Model file for the job. Use its own axes, mm. A direction names the side the tool comes from. Round coordinates to 2 decimals unless told otherwise and drop trailing zeros. Loops run counter-clockwise (first coordinate to the right, second up) from the corner with the lowest first, then second, coordinate; pieces in that order, holes last. Notation, with made-up numbers: (-14.5, 58.5) -> (-3.5, 58.5) arc R20 cw to (-3.5, 91.5) -> close; hole circle Ø10 at (-36.75, 65.5). An arc over 180 degrees is marked (long way). Use a Markdown table: item, result.
from build123d import *

# Parameters (mm, degrees)
SKETCH1_W                         = 152.4
SKETCH1_H                         = 88.9
BASE_FLANGE1_DEPTH                = 1.29032
EDGE_FLANGE1_STRIP_W              = 5.85978
EDGE_FLANGE1_STRIP_H              = 1.29032
EDGE_FLANGE1_STRIP_CUT_DEPTH      = 88.9
EDGE_FLANGE1_STRIP_2_W            = 5.85978
EDGE_FLANGE1_STRIP_2_H            = 1.29032
EDGE_FLANGE1_STRIP_CUT_2_DEPTH    = 88.9
EDGE_FLANGE1_DEPTH                = 88.9
EDGE_FLANGE1_BEND_DEPTH           = 88.9
F_4_22MM_HOLE_FOR_M3_CLINCH_NUT_D = 4.22
BREAK_CORNER1_START               = -77.68082
BREAK_CORNER1_DEPTH               = 155.36164
CUT_THICKEN1_START                = 41.91
CUT_THICKEN1_OUTLINE_W            = 0.127
CUT_THICKEN1_OUTLINE_H            = 1.29032
CUT_THICKEN1_DEPTH                = 2.54
CUT_THICKEN2_START                = 41.91
CUT_THICKEN2_OUTLINE_W            = 0.127
CUT_THICKEN2_OUTLINE_H            = 1.29032
CUT_THICKEN2_DEPTH                = 2.54
MIRROR7_START                     = 41.91
MIRROR7_COPY_1_SKETCH_W           = 0.127
MIRROR7_COPY_1_SKETCH_H           = 1.29032
MIRROR7_COPY_1_DEPTH              = 2.54
MIRROR7_COPY_2_SKETCH_W           = 0.127
MIRROR7_COPY_2_SKETCH_H           = 1.29032
MIRROR7_COPY_2_DEPTH              = 2.54
MOVE_FACE1_BY                     = 1.27
MOVE_FACE1_2_BY                   = 1.27
MOVE_FACE1_3_BY                   = 1.27
MOVE_FACE1_4_BY                   = 1.27
EDGE_FLANGE2_STRIP_W              = 5.66928
EDGE_FLANGE2_STRIP_H              = 1.29032
EDGE_FLANGE2_STRIP_CUT_DEPTH      = 2.54
EDGE_FLANGE2_STRIP_2_W            = 5.66928
EDGE_FLANGE2_STRIP_2_H            = 1.29032
EDGE_FLANGE2_STRIP_CUT_2_DEPTH    = 2.54
EDGE_FLANGE2_STRIP_3_W            = 5.66928
EDGE_FLANGE2_STRIP_3_H            = 1.29032
EDGE_FLANGE2_STRIP_CUT_3_DEPTH    = 2.54
EDGE_FLANGE2_STRIP_4_W            = 5.66928
EDGE_FLANGE2_STRIP_4_H            = 1.29032
EDGE_FLANGE2_STRIP_CUT_4_DEPTH    = 2.54
EDGE_FLANGE2_DEPTH                = 2.54
EDGE_FLANGE2_BEND_DEPTH           = 2.54
EDGE_FLANGE2_BEND_2_DEPTH         = 2.54
EDGE_FLANGE2_BEND_3_DEPTH         = 2.54


# Read off the part's stored shape, not the designer's step: Break-Corner1, Cut-Thicken1, Cut-Thicken2
# Sheet-metal steps are written as plain solids
with BuildPart() as part:
    # Sketch1 → Base-Flange1 (new body)
    with BuildSketch(Plane.XY):
        Rectangle(SKETCH1_W, SKETCH1_H)
    extrude(amount=-BASE_FLANGE1_DEPTH)

    # Edge-Flange1 strip (across the edge) → Edge-Flange1 strip cut (cut)
    with BuildSketch(Plane(origin=(-76.3905, -44.45, -1.29032), x_dir=(1, 0, 0), z_dir=(0, 1, 0))):
        with Locations((-2.67589, -0.64516)):
            Rectangle(EDGE_FLANGE1_STRIP_W, EDGE_FLANGE1_STRIP_H)
    extrude(amount=EDGE_FLANGE1_STRIP_CUT_DEPTH, mode=Mode.SUBTRACT)

    # Edge-Flange1 strip 2 (across the edge) → Edge-Flange1 strip cut 2 (cut)
    with BuildSketch(Plane(origin=(76.3905, 44.45, -1.29032), x_dir=(-1, 0, 0), z_dir=(0, -1, 0))):
        with Locations((-2.67589, -0.64516)):
            Rectangle(EDGE_FLANGE1_STRIP_2_W, EDGE_FLANGE1_STRIP_2_H)
    extrude(amount=EDGE_FLANGE1_STRIP_CUT_2_DEPTH, mode=Mode.SUBTRACT)

    # Edge-Flange1 section (across the edge) → Edge-Flange1 (add)
    with BuildSketch(Plane(origin=(-76.3905, -44.45, -1.29032), x_dir=(1, 0, 0), z_dir=(0, 1, 0))):
        with BuildLine():
            Line((-1.29032, 0.254), (-1.29032, 46.96968))
            Line((-1.29032, 46.96968), (0, 46.96968))
            Line((0, 46.96968), (0, 0.254))
            ThreePointArc((0, 0.254), (0.074394878, 0.074394878), (0.254, 0))
            Line((0.254, 0), (0.254, -1.29032))
            ThreePointArc((0.254, -1.29032), (-0.837999144, -0.837999144), (-1.29032, 0.254))
        make_face()
    extrude(amount=EDGE_FLANGE1_DEPTH)

    # Edge-Flange1 section 2 (across the edge) → Edge-Flange1 bend (add)
    with BuildSketch(Plane(origin=(76.3905, 44.45, -1.29032), x_dir=(-1, 0, 0), z_dir=(0, -1, 0))):
        with BuildLine():
            Line((-1.29032, 0.254), (-1.29032, 46.96968))
            Line((-1.29032, 46.96968), (0, 46.96968))
            Line((0, 46.96968), (0, 0.254))
            ThreePointArc((0, 0.254), (0.074394878, 0.074394878), (0.254, 0))
            Line((0.254, 0), (0.254, -1.29032))
            ThreePointArc((0.254, -1.29032), (-0.837999144, -0.837999144), (-1.29032, 0.254))
        make_face()
    extrude(amount=EDGE_FLANGE1_BEND_DEPTH)

    # Ø4.22mm hole for M3 Clinch nut (through all)
    with Locations(Plane.ZY.offset(77.68082)):
        with Locations((-43.26, 0)):
            f_4_22mm_hole_for_m3_clinch_nut = Hole(F_4_22MM_HOLE_FOR_M3_CLINCH_NUT_D / 2)

    # Mirror1: Ø4.22mm hole for M3 Clinch nut across plane
    add(f_4_22mm_hole_for_m3_clinch_nut.mirror(Plane(origin=(0, 0, 0), x_dir=(0, 0, 1), z_dir=(1, 0, 0))), mode=Mode.SUBTRACT)

    # Break-Corner1 outline → Break-Corner1 (cut)
    with BuildSketch(Plane.YZ.offset(BREAK_CORNER1_START)):
        with BuildLine():
            Line((44.45, -48.26), (44.45, -48.006))
            ThreePointArc((44.45, -48.006), (44.375605122, -48.185605122), (44.196, -48.26))
            Line((44.196, -48.26), (44.45, -48.26))
        make_face()
        with BuildLine():
            Line((-44.45, -48.26), (-44.196, -48.26))
            ThreePointArc((-44.196, -48.26), (-44.375605122, -48.185605122), (-44.45, -48.006))
            Line((-44.45, -48.006), (-44.45, -48.26))
        make_face()
    extrude(amount=BREAK_CORNER1_DEPTH, mode=Mode.SUBTRACT)

    # Cut-Thicken1 outline → Cut-Thicken1 (cut)
    with BuildSketch(Plane(origin=(0, 0, 0), x_dir=(1, 0, 0), z_dir=(0, 1, 0)).offset(CUT_THICKEN1_START)):
        with Locations((36.97732, 0.64516)):
            Rectangle(CUT_THICKEN1_OUTLINE_W, CUT_THICKEN1_OUTLINE_H)
    cut_thicken1 = extrude(amount=CUT_THICKEN1_DEPTH, mode=Mode.SUBTRACT)

    # Cut-Thicken2 outline → Cut-Thicken2 (cut)
    with BuildSketch(Plane(origin=(0, 0, 0), x_dir=(1, 0, 0), z_dir=(0, 1, 0)).offset(CUT_THICKEN2_START)):
        with Locations((39.64432, 0.64516)):
            Rectangle(CUT_THICKEN2_OUTLINE_W, CUT_THICKEN2_OUTLINE_H)
    cut_thicken2 = extrude(amount=CUT_THICKEN2_DEPTH, mode=Mode.SUBTRACT)

    # Mirror6: Cut-Thicken1, Cut-Thicken2 across plane
    add(cut_thicken1.mirror(Plane(origin=(0, 0, 0), x_dir=(0, 0, 1), z_dir=(1, 0, 0))), mode=Mode.SUBTRACT)
    add(cut_thicken2.mirror(Plane(origin=(0, 0, 0), x_dir=(0, 0, 1), z_dir=(1, 0, 0))), mode=Mode.SUBTRACT)

    # Mirror7: Cut-Thicken1, Cut-Thicken2 across plane
    add(cut_thicken1.mirror(Plane.ZX), mode=Mode.SUBTRACT)
    add(cut_thicken2.mirror(Plane.ZX), mode=Mode.SUBTRACT)

    # Mirror7 copy 1 sketch → Mirror7 copy 1 (cut)
    with BuildSketch(Plane(origin=(0, 0, 0), x_dir=(-1, 0, 0), z_dir=(0, -1, 0)).offset(MIRROR7_START)):
        with Locations((36.97732, 0.64516)):
            Rectangle(MIRROR7_COPY_1_SKETCH_W, MIRROR7_COPY_1_SKETCH_H)
    extrude(amount=MIRROR7_COPY_1_DEPTH, mode=Mode.SUBTRACT)

    # Mirror7 copy 2 sketch → Mirror7 copy 2 (cut)
    with BuildSketch(Plane(origin=(0, 0, 0), x_dir=(-1, 0, 0), z_dir=(0, -1, 0)).offset(MIRROR7_START)):
        with Locations((39.64432, 0.64516)):
            Rectangle(MIRROR7_COPY_2_SKETCH_W, MIRROR7_COPY_2_SKETCH_H)
    extrude(amount=MIRROR7_COPY_2_DEPTH, mode=Mode.SUBTRACT)

    # Move Face1: a face moved inward by 1.27
    extrude(part.faces().sort_by_distance((-38.31082, -44.45, -0.64516))[0], amount=MOVE_FACE1_BY, dir=(0, 1, 0), mode=Mode.SUBTRACT)

    # Move Face1 2: a face moved inward by 1.27
    extrude(part.faces().sort_by_distance((38.31082, -44.45, -0.64516))[0], amount=MOVE_FACE1_2_BY, dir=(0, 1, 0), mode=Mode.SUBTRACT)

    # Move Face1 3: a face moved inward by 1.27
    extrude(part.faces().sort_by_distance((-38.31082, 44.45, -0.64516))[0], amount=MOVE_FACE1_3_BY, dir=(0, -1, 0), mode=Mode.SUBTRACT)

    # Move Face1 4: a face moved inward by 1.27
    extrude(part.faces().sort_by_distance((38.31082, 44.45, -0.64516))[0], amount=MOVE_FACE1_4_BY, dir=(0, -1, 0), mode=Mode.SUBTRACT)

    # Edge-Flange2 strip (across the edge) → Edge-Flange2 strip cut (cut)
    with BuildSketch(Plane(origin=(37.04082, 43.18, -1.29032), x_dir=(0, -1, 0), z_dir=(1, 0, 0))):
        with Locations((-1.29032, -0.64516)):
            Rectangle(EDGE_FLANGE2_STRIP_W, EDGE_FLANGE2_STRIP_H)
    extrude(amount=EDGE_FLANGE2_STRIP_CUT_DEPTH, mode=Mode.SUBTRACT)

    # Edge-Flange2 strip 2 (across the edge) → Edge-Flange2 strip cut 2 (cut)
    with BuildSketch(Plane(origin=(-39.58082, 43.18, -1.29032), x_dir=(0, -1, 0), z_dir=(1, 0, 0))):
        with Locations((-1.29032, -0.64516)):
            Rectangle(EDGE_FLANGE2_STRIP_2_W, EDGE_FLANGE2_STRIP_2_H)
    extrude(amount=EDGE_FLANGE2_STRIP_CUT_2_DEPTH, mode=Mode.SUBTRACT)

    # Edge-Flange2 strip 3 (across the edge) → Edge-Flange2 strip cut 3 (cut)
    with BuildSketch(Plane(origin=(39.58082, -43.18, -1.29032), x_dir=(0, 1, 0), z_dir=(-1, 0, 0))):
        with Locations((-1.29032, -0.64516)):
            Rectangle(EDGE_FLANGE2_STRIP_3_W, EDGE_FLANGE2_STRIP_3_H)
    extrude(amount=EDGE_FLANGE2_STRIP_CUT_3_DEPTH, mode=Mode.SUBTRACT)

    # Edge-Flange2 strip 4 (across the edge) → Edge-Flange2 strip cut 4 (cut)
    with BuildSketch(Plane(origin=(-37.04082, -43.18, -1.29032), x_dir=(0, 1, 0), z_dir=(-1, 0, 0))):
        with Locations((-1.29032, -0.64516)):
            Rectangle(EDGE_FLANGE2_STRIP_4_W, EDGE_FLANGE2_STRIP_4_H)
    extrude(amount=EDGE_FLANGE2_STRIP_CUT_4_DEPTH, mode=Mode.SUBTRACT)

    # Edge-Flange2 section (across the edge) → Edge-Flange2 (add)
    with BuildSketch(Plane(origin=(37.04082, 43.18, -1.29032), x_dir=(0, -1, 0), z_dir=(1, 0, 0))):
        with BuildLine():
            Line((0, 0.254), (0, 1.27))
            Line((0, 1.27), (1.29032, 1.27))
            Line((1.29032, 1.27), (1.29032, 0.254))
            ThreePointArc((1.29032, 0.254), (1.364714878, 0.074394878), (1.54432, 0))
            Line((1.54432, 0), (1.54432, -1.29032))
            ThreePointArc((1.54432, -1.29032), (0.452320856, -0.837999144), (0, 0.254))
        make_face()
    extrude(amount=EDGE_FLANGE2_DEPTH)

    # Edge-Flange2 section 2 (across the edge) → Edge-Flange2 bend (add)
    with BuildSketch(Plane(origin=(-39.58082, 43.18, -1.29032), x_dir=(0, -1, 0), z_dir=(1, 0, 0))):
        with BuildLine():
            Line((0, 0.254), (0, 1.27))
            Line((0, 1.27), (1.29032, 1.27))
            Line((1.29032, 1.27), (1.29032, 0.254))
            ThreePointArc((1.29032, 0.254), (1.364714878, 0.074394878), (1.54432, 0))
            Line((1.54432, 0), (1.54432, -1.29032))
            ThreePointArc((1.54432, -1.29032), (0.452320856, -0.837999144), (0, 0.254))
        make_face()
    extrude(amount=EDGE_FLANGE2_BEND_DEPTH)

    # Edge-Flange2 section 3 (across the edge) → Edge-Flange2 bend 2 (add)
    with BuildSketch(Plane(origin=(39.58082, -43.18, -1.29032), x_dir=(0, 1, 0), z_dir=(-1, 0, 0))):
        with BuildLine():
            Line((0, 0.254), (0, 1.27))
            Line((0, 1.27), (1.29032, 1.27))
            Line((1.29032, 1.27), (1.29032, 0.254))
            ThreePointArc((1.29032, 0.254), (1.364714878, 0.074394878), (1.54432, 0))
            Line((1.54432, 0), (1.54432, -1.29032))
            ThreePointArc((1.54432, -1.29032), (0.452320856, -0.837999144), (0, 0.254))
        make_face()
    extrude(amount=EDGE_FLANGE2_BEND_2_DEPTH)

    # Edge-Flange2 section 4 (across the edge) → Edge-Flange2 bend 3 (add)
    with BuildSketch(Plane(origin=(-37.04082, -43.18, -1.29032), x_dir=(0, 1, 0), z_dir=(-1, 0, 0))):
        with BuildLine():
            Line((0, 0.254), (0, 1.27))
            Line((0, 1.27), (1.29032, 1.27))
            Line((1.29032, 1.27), (1.29032, 0.254))
            ThreePointArc((1.29032, 0.254), (1.364714878, 0.074394878), (1.54432, 0))
            Line((1.54432, 0), (1.54432, -1.29032))
            ThreePointArc((1.54432, -1.29032), (0.452320856, -0.837999144), (0, 0.254))
        make_face()
    extrude(amount=EDGE_FLANGE2_BEND_3_DEPTH)


solid = part.part
Q1. Flat gauge pins, fed straight in: pin 1 (0.6 mm diameter, centred on y = -43, z = -1, fed in from +X); pin 2 (8 mm diameter, centred on x = 53, y = 14.5, fed in from -Z); pin 3 (3 mm diameter, centred on x = -1, y = -14, fed in from +Z); pin 4 (1.1 mm diameter, centred on x = 39, z = -2, fed in from -Y). Where does each tip first touch, or does it go through?
Results list:
| item | result |
|---|---|
| pin 1 | stops at x = 77.66 |
| pin 2 | stops at z = -1.29 |
| pin 3 | stops at z = 0 |
| pin 4 | stops at y = -43.18 |
Q2. Drill centre lines: L1, parallel to X at y = -14, z = -14.5; L2, parallel to Y at x = -76.85, z = -43.26; L3, parallel to Z at x = 45, y = 1. Where is each one in solid material? Low to high. Write a range as from..to.
Results list:
| item | result |
|---|---|
| L1 | x = -77.68..-76.39, 76.39..77.68 |
| L2 | y = -44.45..-2.11, 2.11..44.45 |
| L3 | z = -1.29..0 |
Q3. Band-saw the part on A-A, the plane z = -43.26. Give the cut face in (x, y), plus the area to 3 significant figures.
Results list:
| item | result |
|---|---|
| outline | (-77.68, -44.45) -> (-76.39, -44.45) -> (-76.39, -2.11) -> (-77.68, -2.11) -> close; (-77.68, 2.11) -> (-76.39, 2.11) -> (-76.39, 44.45) -> (-77.68, 44.45) -> close; (76.39, -44.45) -> (77.68, -44.45) -> (77.68, -2.11) -> (76.39, -2.11) -> close; (76.39, 2.11) -> (77.68, 2.11) -> (77.68, 44.45) -> (76.39, 44.45) -> close |
| area | 219 mm² |
Q4. Band-saw the part on B-B, the plane y = 0. Give the cut face in (x, z).
Results list:
| item | result |
|---|---|
| outline | (-77.68, -48.26) -> (-76.39, -48.26) -> (-76.39, -45.37) -> (-77.68, -45.37) -> close; (-77.68, -41.15) -> (-76.39, -41.15) -> (-76.39, -1.54) arc R0.25 cw to (-76.14, -1.29) -> (76.14, -1.29) arc R0.25 cw to (76.39, -1.54) -> (76.39, -41.15) -> (77.68, -41.15) -> (77.68, -1.54) arc R1.54 ccw to (76.14, 0) -> (-76.14, 0) arc R1.54 ccw to (-77.68, -1.54) -> close; (76.39, -48.26) -> (77.68, -48.26) -> (77.68, -45.37) -> (76.39, -45.37) -> close |
Q5. Tool access for faces 4 (the face through (76.39, 1, -25)), 5 (the face through (-77, -44.45, -13)): list every direction of +Z, -Z, +X, -X, +Y, -Y with a clear straight run to the whole face (end or side of a thin tool).
Results list:
| item | result |
|---|---|
| face 4 | -Z, +Y, -Y |
| face 5 | +Z, -Z, +X, -X, -Y |
Q6. Band-saw the part on C-C, the plane x = 52. Give the cut face in (y, z), plus the area to 3 significant figures.
Results list:
| item | result |
|---|---|
| outline | (-44.45, -1.29) -> (44.45, -1.29) -> (44.45, 0) -> (-44.45, 0) -> close |
| area | 115 mm² |
Q7. Pull direction Z, two halves, no side cores. Call faces 1 (the face through (77, -44.45, -13)), 2 (the face through (-77.03, 0.09, -41.15)), 3 (the face through (-1, 1, -1.29)): released by +Z, released by -Z, zero draft, split by the parting line, or undercut.
Results list:
| item | result |
|---|---|
| face 1 | zero draft |
| face 2 | undercut |
| face 3 | released by -Z |
